Design review of the part built by this model. Coordinates are the model's own, in mm. Face numbers are marked on the shaded views. A direction names the side the tool comes from. Coordinates: 2 decimals unless noted, no trailing zeros. Write each loop counter-clockwise with the first axis right and the second up, starting at its lowest first coordinate (ties: lowest second). Pieces come first, ordered by that corner, then holes. Notation, with made-up numbers: (62, -32.5) -> (116, -32.5) arc R17 ccw to (116, -28.5) -> close; hole circle Ø11 at (60, -35.75). An arc over 180 degrees is marked (long way). Answer in a Markdown table with one row per item. Add a question column.
Item 1: For the marked faces 4, 5 and 6, list the 3-axis set-ups (+Z, -Z, +X, -X, +Y, -Y) from which the entire face can be reached by the end or side of a thin tool; tool diameter is ignored.
Item 2: Clearance check with flat-ended pins moving along their axes: P1, Ø1.5, axis at y = 31, z = 3.5, coming from the -X side; P2, Ø0.5, axis at x = -2, z = 3, coming from the -Y side; P3, Ø1.6, axis at x = -1.8, z = 3, coming from the +Y side. State where each tip first meets the part, or that it passes through.
Item 3: To check wall thickness, follow line 1 (X direction, y = 29, z = 3); line 2 (Y direction, x = 0.75, z = 3.75); line 3 (X direction, y = 27.25, z = 3). State the ranges of each line that lie inside material, in increasing order.
Item 4: Take a section at A-A, the plane z = 3. Write out the cut boundary in (x, y), and give its area (3 significant figures).
Item 5: Take a section at B-B, the plane z = 1. Write out the cut boundary in (x, y).
Item 6: Draft analysis for pull direction X (two halves, no side actions). For the marked faces 1, 2 and 3, state which applies: released by +X, released by -X, zero draft, split by the parting line, or undercut.
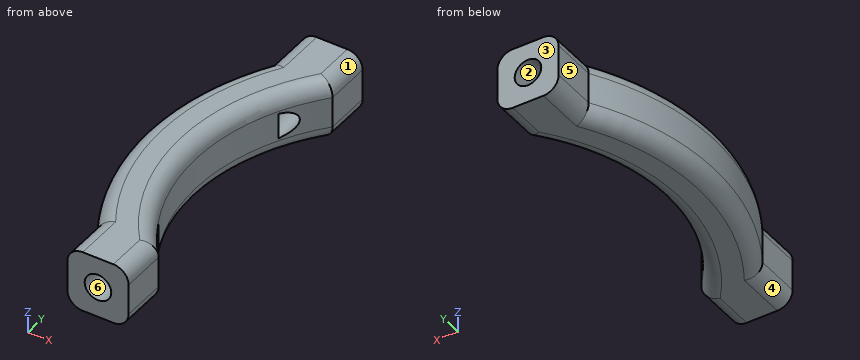
from build123d import *

# Parameters (mm, degrees)
SKETCH1_W             = 6
SKETCH1_H             = 4.5
BOSS_EXTRUDE1_DEPTH   = 6
HOLE1_D               = 2.6
HOLE1_DEPTH           = 8.5
HOLE1_ON_FACE_2_D     = 2.6
HOLE1_ON_FACE_2_DEPTH = 8.5
FILLET1_R             = 1.5


with BuildPart() as part:
    # Sketch1 → Boss-Extrude1 (new body)
    with BuildSketch(Plane.XY):
        with BuildLine():
            Line((1.198715271, 28.132291187), (-4.801284729, 28.132291187))
            ThreePointArc((-4.801284729, 28.132291187), (-8.469932757, 15.132291187), (-4.801284729, 2.132291187))
            Line((-4.801284729, 2.132291187), (1.198715271, 2.132291187))
            ThreePointArc((1.198715271, 2.132291187), (-3.602600575, 15.132291187), (1.198715271, 28.132291187))
        make_face()
        with Locations((-1.801284729, 30.382291187)):
            Rectangle(SKETCH1_W, SKETCH1_H)
        with Locations((-1.801284729, -0.117708813)):
            Rectangle(SKETCH1_W, SKETCH1_H)
    extrude(amount=BOSS_EXTRUDE1_DEPTH)

    # Hole1
    with Locations(Plane(origin=(-1.801284729, 32.632291187, 3), x_dir=(0, 0, 1), z_dir=(0, 1, 0))):
        with Locations((0, 0)):
            Hole(HOLE1_D / 2, depth=HOLE1_DEPTH)

    # Hole1 on face 2
    with Locations(Plane(origin=(-1.801284729, -2.367708813, 3), x_dir=(0, 0, -1), z_dir=(0, -1, 0))):
        with Locations((0, 0)):
            Hole(HOLE1_ON_FACE_2_D / 2, depth=HOLE1_ON_FACE_2_DEPTH)

    # Fillet1
    fillet1_edges = [part.edges().sort_by_distance(p)[0] for p in [
        (1.198715271, 30.382291187, 6),
        (-4.801284729, -0.117708813, 0),
        (-8.469932757, 15.132291187, 0),
        (-4.801284729, 30.382291187, 0),
        (1.198715271, 30.382291187, 0),
        (-3.602600575, 15.132291187, 0),
        (-4.801284729, 30.382291187, 6),
        (-8.469932757, 15.132291187, 6),
        (-4.801284729, -0.117708813, 6),
        (1.198715271, -0.117708813, 6),
        (-3.602600575, 15.132291187, 6),
        (1.198715271, -0.117708813, 0),
    ]]
    fillet(fillet1_edges, radius=FILLET1_R)


solid = part.part
Answers:
| question | item | result |
|---|---|---|
| 1 | face 4 | -Z, -X, -Y |
| 1 | face 5 | +Z, -Z, -X, +Y |
| 1 | face 6 | -Y |
| 2 | P1 | stops at x = -4.8 |
| 2 | P2 | stops at y = 6.13 |
| 2 | P3 | stops at y = 24.13 |
| 3 | line 1 | x = -4.8 to -3.1, -0.5 to 1.2 |
| 3 | line 2 | y = -2.37 to 2.68, 27.59 to 32.63 |
| 3 | line 3 | x = -5.32 to -3.1, -0.5 to 0.49 |
| 4 | outline | (-4.8, -2.37) -> (-3.1, -2.37) -> (-3.1, 6.13) -> (-1.46, 6.13) arc R20 cw to (-1.46, 24.13) -> (-3.1, 24.13) -> (-3.1, 32.63) -> (-4.8, 32.63) -> (-4.8, 28.13) arc R24.87 ccw to (-4.8, 2.13) -> close; (-0.5, -2.37) -> (1.2, -2.37) -> (1.2, 2.13) arc R20 cw to (-0.5, 4.43) -> close; (-0.5, 25.83) arc R20 cw to (1.2, 28.13) -> (1.2, 32.63) -> (-0.5, 32.63) -> close |
| 4 | area | 147 mm^2 |
| 5 | outline | (-4.72, -2.37) -> (1.11, -2.37) -> (1.11, 2.1) arc R20.09 cw to (1.11, 28.16) -> (1.11, 32.63) -> (-4.72, 32.63) -> (-4.72, 28.11) arc R24.78 ccw to (-4.72, 2.16) -> close |
| 6 | face 1 | released by +X |
| 6 | face 2 | undercut |
| 6 | face 3 | zero draft |
